Can you work these out from the model? Positions are in its coordinate system, mm. A direction names the side the tool comes from. Round coordinates to 2 decimals unless told otherwise and drop trailing zeros. Order: outer loops, then holes, each group sorted by start corner. A loop starts at its lowest first (then second) coordinate and runs counter-clockwise, first axis right, second up. Notation, with made-up numbers: (88.5, -15) - (131.5, -15) arc R16 ccw to (131.5, 14) - close; hole circle Ø7 at (-2.5, 72). An arc over 180 degrees is marked (long way). Write item = value, one per line.
from build123d import *

# Parameters (mm, degrees)
F1_DEPTH    = 3
F2_DEPTH    = 1.5
F3_T1_DEPTH = 16.0790165437
F4_SIZE     = 1.49999
F5_T1_DEPTH = 8.1382032795
F5_T4_ANGLE = 209.6600935854
F5_T6_ANGLE = 209.6600935854


# Not quite as in the source:
# - a fillet or chamfer that OpenCascade refuses, or shapes differently, is made with other operations: its cross-section is extruded or revolved along the edge and cut away or added
# - a fillet or chamfer is up to 0.001 mm smaller than in the source, because OpenCascade refuses the exact size


with BuildPart() as f1:
    # F0 (on Top) → F1 (new body)
    with BuildSketch(Plane.XY):
        with BuildLine():
            Line((-17.480337616, -3.0822551536), (-15.0183182334, -2.6481347094))
            ThreePointArc((-15.0183182334, -2.6481347094), (0, 15.25), (15.0183182334, -2.6481347094))
            Line((15.0183182334, -2.6481347094), (17.480337616, -3.0822551536))
            ThreePointArc((17.480337616, -3.0822551536), (0, 17.75), (-17.480337616, -3.0822551536))
        make_face()
    extrude(amount=F1_DEPTH)

    # F0 (on Top) → F2 (join)
    with BuildSketch(Plane.XY):
        with BuildLine():
            Line((-17.480337616, -3.0822551536), (-15.0183182334, -2.6481347094))
            ThreePointArc((-15.0183182334, -2.6481347094), (0, 15.25), (15.0183182334, -2.6481347094))
            Line((15.0183182334, -2.6481347094), (17.480337616, -3.0822551536))
            ThreePointArc((17.480337616, -3.0822551536), (0, 17.75), (-17.480337616, -3.0822551536))
        make_face()
        with BuildLine():
            Line((-15.0183182334, -2.6481347094), (-4.5, -0.7934714132))
            ThreePointArc((-4.5, -0.7934714132), (0, 4.5694197535), (4.5, -0.7934714132))
            Line((4.5, -0.7934714132), (15.0183182334, -2.6481347094))
            ThreePointArc((15.0183182334, -2.6481347094), (0, 15.25), (-15.0183182334, -2.6481347094))
        make_face()
        with BuildLine():
            Line((-5.5861435714, 7.8488852712), (-4.5254833996, 6.7882250994))
            ThreePointArc((-4.5254833996, 6.7882250994), (-4.5254833996, 4.5254833996), (-6.7882250994, 4.5254833996))
            Line((-6.7882250994, 4.5254833996), (-7.8488852712, 5.5861435714))
            ThreePointArc((-7.8488852712, 5.5861435714), (-7.8488852712, 7.8488852712), (-5.5861435714, 7.8488852712))
        make_face(mode=Mode.SUBTRACT)
        with BuildLine():
            ThreePointArc((6.7882250994, 4.5254833996), (4.5254833996, 4.5254833996), (4.5254833996, 6.7882250994))
            Line((4.5254833996, 6.7882250994), (5.5861435714, 7.8488852712))
            ThreePointArc((5.5861435714, 7.8488852712), (7.8488852712, 7.8488852712), (7.8488852712, 5.5861435714))
            Line((7.8488852712, 5.5861435714), (6.7882250994, 4.5254833996))
        make_face(mode=Mode.SUBTRACT)
    extrude(amount=-F2_DEPTH)

    # F3: chamfer of 2 on 2 edges, made by hand

    # F3_s2 → F3_t1 (cut)
    with BuildSketch(Plane.XY.offset(-7.2895082718)):
        with BuildLine():
            Line((-15.3851589244, -2.7128186209), (-17.7302273788, -0.8375781136))
            ThreePointArc((-17.7302273788, -0.8375781136), (-17.6441291813, -1.935769985), (-17.480337616, -3.0822551536))
            Line((-17.480337616, -3.0822551536), (-15.3851589244, -2.7128186209))
        make_face()
        with BuildLine():
            Line((15.3851589244, -2.7128186209), (17.7302273788, -0.8375781136))
            ThreePointArc((17.7302273788, -0.8375781136), (17.6441291813, -1.935769985), (17.480337616, -3.0822551536))
            Line((17.480337616, -3.0822551536), (15.3851589244, -2.7128186209))
        make_face()
    extrude(amount=F3_T1_DEPTH, mode=Mode.SUBTRACT)

    # F4 (size 1.5 in the source; OpenCascade refuses exactly that, so slightly less here)
    f4_edges = [f1.edges().sort_by_distance(p)[0] for p in [
        (9.942579, -1.753145, -1.5),
        (-9.942579, -1.753145, -1.5),
    ]]
    chamfer(f4_edges, length=F4_SIZE)

    # F5: fillet of radius 1.5 on 4 edges, made by hand

    # F5_s2 → F5_t1 (cut)
    with BuildSketch(Plane.XY.offset(-3.3191016398)):
        with BuildLine():
            ThreePointArc((-17.7496579301, -0.1101969358), (-17.5995489023, -0.7550040841), (-17.1864813575, -1.2723861308))
            Line((-17.1864813575, -1.2723861308), (-17.7302273788, -0.8375781136))
            ThreePointArc((-17.7302273788, -0.8375781136), (-17.7436703144, -0.4739871018), (-17.7496579301, -0.1101969358))
        make_face()
        with BuildLine():
            ThreePointArc((17.1864813575, -1.2723861308), (17.5995489023, -0.7550040841), (17.7496579301, -0.1101969358))
            ThreePointArc((17.7496579301, -0.1101969358), (17.7436703144, -0.4739871018), (17.7302273788, -0.8375781136))
            Line((17.7302273788, -0.8375781136), (17.1864813575, -1.2723861308))
        make_face()
    extrude(amount=F5_T1_DEPTH, mode=Mode.SUBTRACT)

    # F5_s3 → F5_t4 (revolve, cut)
    with BuildSketch(Plane(origin=(0, 0, 0), x_dir=(0, 0, 1), z_dir=(-0.2559527399, -0.966689296, 0))):
        with BuildLine():
            ThreePointArc((3, -16.25), (2.5606601718, -17.3106601718), (1.5, -17.75))
            Line((1.5, -17.75), (3, -17.75))
            Line((3, -17.75), (3, -16.25))
        make_face()
    revolve(axis=Axis((0, 0, 3), (0, 0, 1)), revolution_arc=F5_T4_ANGLE, mode=Mode.SUBTRACT)

    # F5_s5 → F5_t6 (revolve, cut)
    with BuildSketch(Plane(origin=(0, 0, 0), x_dir=(0, 0, 1), z_dir=(-0.2559527399, -0.966689296, 0))):
        with BuildLine():
            ThreePointArc((-1.5, -16.25), (-1.0606601718, -17.3106601718), (0, -17.75))
            Line((0, -17.75), (-1.5, -17.75))
            Line((-1.5, -17.75), (-1.5, -16.25))
        make_face()
    revolve(axis=Axis((0, 0, -1.5), (0, 0, 1)), revolution_arc=F5_T6_ANGLE, mode=Mode.SUBTRACT)


solid = f1.part
(1) On a 3-axis mill with a long thin cutter (end or side, diameter ignored), from which of +Z, -Z, +X, -X, +Y, -Y can I reach the whole of each face in a straight line? I mean faces 4 (the face through (-5.063, 7.326, -0.74)), 5 (the face through (-0.373, 15.245, 1.479)), 6 (the face through (2.33, 15.24, 3)). Say none if no direction works.
Computed:
face_4 = +Z, -Z
face_5 = +Z
face_6 = +Z, +X, -X, +Y, -Y
(2) Will these pins go through, and if not, where does the flat tip stop? P1, Ø2, axis at y = 15.5, z = 0.5, coming from the +X side; P2, Ø1.5, axis at y = 2.5, z = 0.5, coming from the -X side.
Computed:
P1 = 10.24
P2 = -17.66
(3) Thinking about a two-plate mould opening in Y: for faces 1 (the face through (0, 8, -1.5)), 2 (the face through (16.273, -2.003, 0.788)), 3 (the face through (7.326, 5.063, -0.74)), which applies, +Y half, -Y half, draft (parallel to the pull), parting line (faces both ways), or undercut?
Computed:
face_1 = draft
face_2 = -Y half
face_3 = undercut
(4) If I drill on line 1 (X direction, y = 0, z = 1.3); line 2 (Z direction, x = 15, y = -0.25); line 3 (Y direction, x = 0, z = 1.45), over which ranges is the centre line in solid material (lowest first)? Write a range as from..to.
Computed:
line_1 = -17.75..-15.25, 15.25..17.75
line_2 = -1.5..0
line_3 = 15.25..17.75
(5) If we section it at B-B (x = 0): Write out the boundary of the cut face in (y, z).
Computed:
outline = (4.57, -1.5) - (16.25, -1.5) arc R1.5 ccw to (17.75, 0) - (17.75, 1.5) arc R1.5 ccw to (16.25, 3) - (15.25, 3) - (15.25, 0) - (4.57, 0) - close
